Could you check a few things on this model? Use its own coordinates, in mm. Coordinates: 2 decimals unless noted, no trailing zeros. Loops run counter-clockwise (first coordinate to the right, second up) from the corner with the lowest first, then second, coordinate; pieces in that order, holes last. Notation, with made-up numbers: M 26,61.25 L 35,61.25 A17 cw 35,71.25 Z; hole C 0,81.25 d3. An arc over 180 degrees is marked long. Write each question's results on one line, items separated by ' | '.
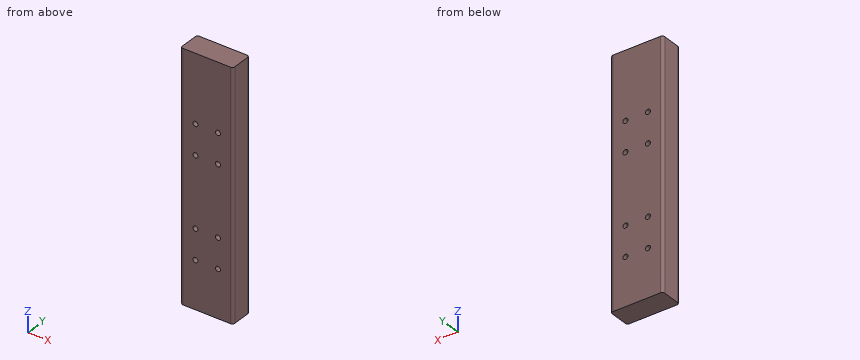
```python
from build123d import *

# Parameters (mm, degrees)
SKETCH1_W           = 42
SKETCH1_H           = 18
BOSS_EXTRUDE1_DEPTH = 196
FILLET1_R           = 2
SKETCH2_R           = 2
CUT_EXTRUDE1_DEPTH  = 202.25605581


with BuildPart() as part:
    # Sketch1 → Boss-Extrude1 (new body)
    with BuildSketch(Plane.XY):
        with Locations((21, 9)):
            Rectangle(SKETCH1_W, SKETCH1_H)
    extrude(amount=BOSS_EXTRUDE1_DEPTH)

    # Fillet1
    fillet1_edges = [part.edges().sort_by_distance(p)[0] for p in [
        (0, 18, 98),
        (42, 18, 98),
        (42, 0, 98),
        (0, 0, 98),
    ]]
    fillet(fillet1_edges, radius=FILLET1_R)

    # Sketch2 → Cut-Extrude1 (cut, through all)
    with BuildSketch(Plane.XZ):
        with Locations(Location((12, 142, 0), (0, 0, 270))):
            Circle(SKETCH2_R)
        with Locations(Location((30, 142, 0), (0, 0, 270))):
            Circle(SKETCH2_R)
        with Locations(Location((12, 118, 0), (0, 0, 270))):
            Circle(SKETCH2_R)
        with Locations(Location((30, 118, 0), (0, 0, 270))):
            Circle(SKETCH2_R)
        with Locations(Location((12, 62, 0), (0, 0, 270))):
            Circle(SKETCH2_R)
        with Locations(Location((30, 62, 0), (0, 0, 270))):
            Circle(SKETCH2_R)
        with Locations(Location((30, 38, 0), (0, 0, 270))):
            Circle(SKETCH2_R)
        with Locations(Location((12, 38, 0), (0, 0, 270))):
            Circle(SKETCH2_R)
    extrude(amount=-CUT_EXTRUDE1_DEPTH, mode=Mode.SUBTRACT)


solid = part.part
```
(1) Imagine slicing it at A-A, the plane z = 118. List the corners of the cut face in (x, y) for me, and give its area (3 significant figures).
Reported:
outline: M 0,2 A2 ccw 2,0 L 10,0 L 10,18 L 2,18 A2 ccw 0,16 Z; M 14,0 L 28,0 L 28,18 L 14,18 Z; M 32,0 L 40,0 A2 ccw 42,2 L 42,16 A2 ccw 40,18 L 32,18 Z | area: 609 mm2
(2) Please list where these lines run through material, in increasing order: probe 1 along X at (y, z) = (7, 118); probe 2 along Z at (x, y) = (31, 11.5); probe 3 along X at (y, z) = (16.25, 178.5). Write a range as from..to.
Reported:
probe 1: x = 0..10, 14..28, 32..42 | probe 2: z = 0..36.27, 39.73..60.27, 63.73..116.27, 119.73..140.27, 143.73..196 | probe 3: x = 0.02..41.98
(3) Will this pin go through, and if not, where does the flat tip stop? P1, Ø2.5, axis at x = 12, z = 142, coming from the +Y side.
Reported:
P1: passes through
(4) Imagine slicing it at B-B, the plane x = 30. List the corners of the cut face in (y, z) for me.
Reported:
outline: M 0,0 L 18,0 L 18,36 L 0,36 Z; M 0,40 L 18,40 L 18,60 L 0,60 Z; M 0,64 L 18,64 L 18,116 L 0,116 Z; M 0,120 L 18,120 L 18,140 L 0,140 Z; M 0,144 L 18,144 L 18,196 L 0,196 Z
